Geometry check sheet. Reference: drawing and pictorial views, mm from the part's lowest x, y, z. Round coordinates to 2 decimals unless told otherwise and drop trailing zeros. Write each loop counter-clockwise with the first axis right and the second up, starting at its lowest first coordinate (ties: lowest second). Pieces come first, ordered by that corner, then holes. Notation, with made-up numbers: M -1.75,-0.5 L 34.25,-0.5 A25 cw 34.25,37.5 Z; hole C 89,-33.75 d6. An arc over 180 degrees is marked long. Put each result on its own line as item: value. Start each with the question number.
(1) Section check D-D on z = 30. Record the cut outline in (x, y).
(2) Section check C-C on y = 1.7. Record the cut outline in (x, z).
(3) Section check A-A on x = 33. Record the cut outline in (y, z).
(4) Section check B-B on z = 56. Record the cut outline in (x, y) (1 decimal).
(5) Material ranges on probe 1 along Z at (x, y) = (22.5, 0.95) (1 decimal); probe 2 along X at (y, z) = (0.55, 55.5) (1 decimal); probe 3 along X at (y, z) = (0.65, 51), recorded low to high.
(6) Gauge pin test, flat ends, axial feed: pin 1 (1 mm diameter, centred on y = 1, z = 38, fed in from -X); pin 2 (14.5 mm diameter, centred on x = 54, z = 33, fed in from +Y). Record the tip position at first contact, or that the pin passes through.
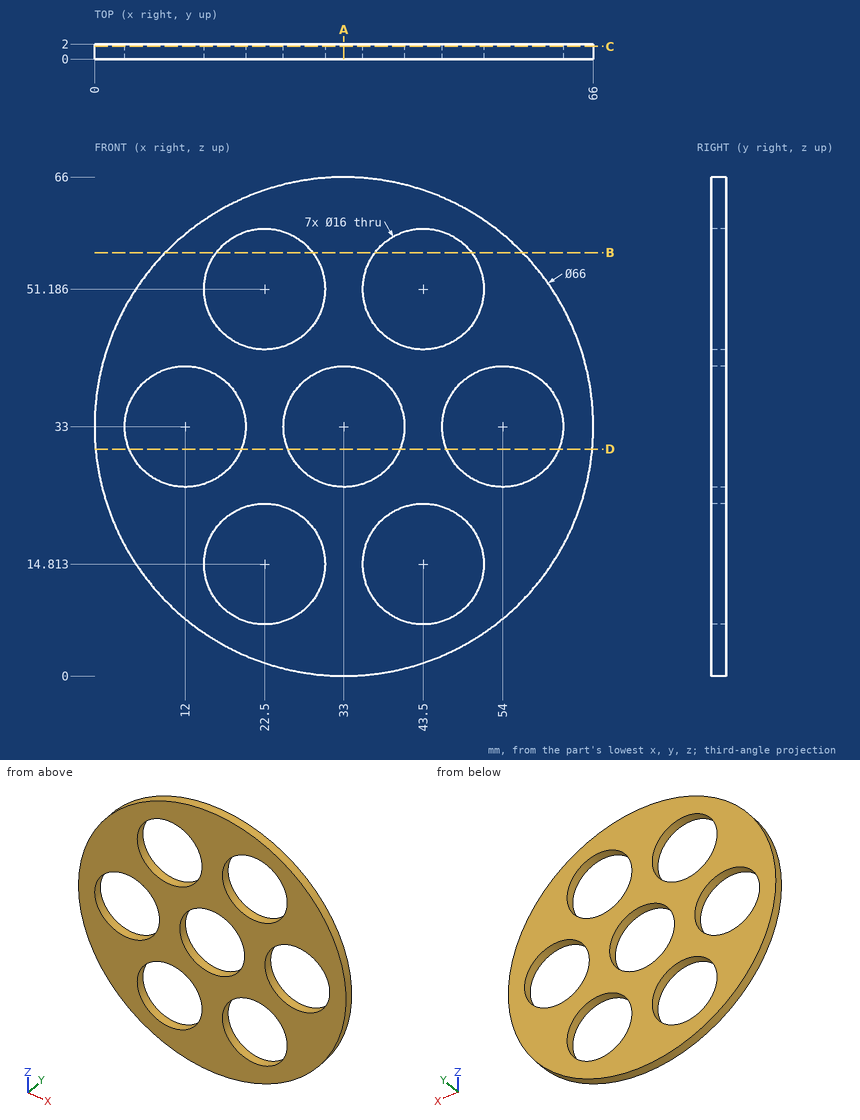
Answers follow:
1. outline: M 0.14,0 L 4.58,0 L 4.58,2 L 0.14,2 Z; M 19.42,0 L 25.58,0 L 25.58,2 L 19.42,2 Z; M 40.42,0 L 46.58,0 L 46.58,2 L 40.42,2 Z; M 61.42,0 L 65.86,0 L 65.86,2 L 61.42,2 Z
2. outline: C 33,33 d66; hole C 12,33 d16; hole C 22.5,14.81 d16; hole C 22.5,51.19 d16; hole C 33,33 d16; hole C 43.5,14.81 d16; hole C 43.5,51.19 d16; hole C 54,33 d16
3. outline: M 0,0 L 2,0 L 2,25 L 0,25 Z; M 0,41 L 2,41 L 2,66 L 0,66 Z
4. outline: M 9.3,0 L 16.1,0 L 16.1,2 L 9.3,2 Z; M 28.9,0 L 37.1,0 L 37.1,2 L 28.9,2 Z; M 49.9,0 L 56.7,0 L 56.7,2 L 49.9,2 Z
5. probe 1: z = 1.7 to 6.8, 22.8 to 43.2, 59.2 to 64.3
5. probe 2: x = 8.9 to 15.8, 29.2 to 36.8, 50.2 to 57.1
5. probe 3: x = 5.34 to 14.5, 30.5 to 35.5, 51.5 to 60.66
6. pin 1: stops at x = 0.31
6. pin 2: passes through
